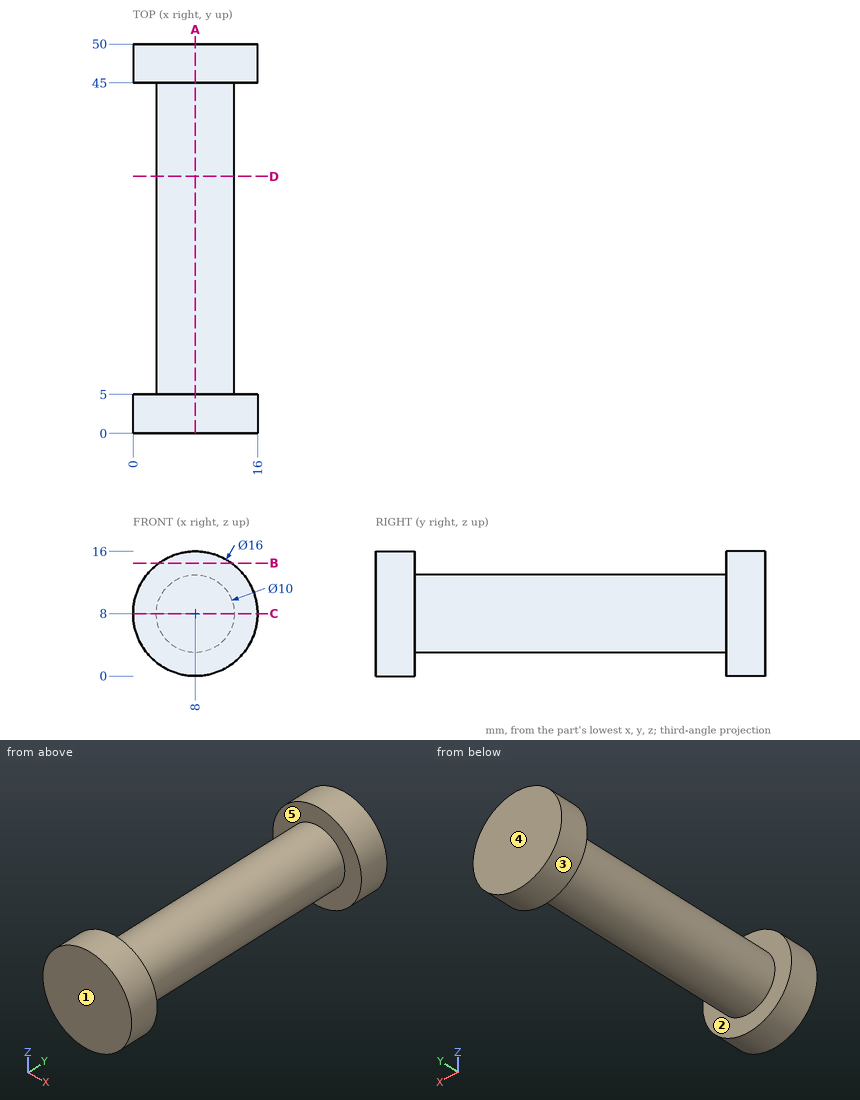
Input: dimensioned drawing with shaded views. Units: mm. Origin: part minimum x, y, z. A direction names the side the tool comes from. Give positions to 0.01 mm unless a question says otherwise; leave off trailing zeros. Loops run counter-clockwise (first coordinate to the right, second up) from the corner with the lowest first, then second, coordinate; pieces in that order, holes last. Notation, with made-up numbers: (84.5, 36) - (90.5, 36) arc R22 cw to (90.5, 61) - close; hole circle Ø6 at (86, -37). An arc over 180 degrees is marked (long way). Answer as CSV lines item,"result". Start each with the question number.
(1) Ray query, line 1 along Y through (x, z) = (15.5, 7); line 2 along X through (y, z) = (17, 12); line 3 along X through (y, z) = (44, 3.5). Return the intervals inside material, ascending. Write a range as [from, to].
(2) Section query C-C (z = 8). Output: boundary loops of the cut face in (x, y).
(3) Reachability of the marked faces 1 and 2 from +Z, -Z, +X, -X, +Y, -Y: full face, straight path, thin tool, end or side. Return the list, or none.
(4) Section query B-B (z = 14.5). Output: boundary loops of the cut face in (x, y).
(5) Section query D-D (y = 33). Output: boundary loops of the cut face in (x, z), and give its area (3 significant figures).
(6) Mould query, pull axis Y, two halves, no side actions, for the marked faces 3, 4 and 5. Classes: +Y half, -Y half, draft (parallel to the pull), parting line (faces both ways), or undercut.
(7) Section query A-A (x = 8). Output: boundary loops of the cut face in (y, z), and give its area (3 significant figures).
(8) Pin query (flat end, axial travel): P1, Ø1, axis at y = 33, z = 12.5, coming from the -X side; P2, Ø6, axis at x = 3, z = 9.5, coming from the -Y side; P3, Ø8, axis at x = 9, y = 36.5, coming from the -Z side; P4, Ø5, axis at y = 38, z = 2.5, coming from the -X side. Return the tip coordinate at first contact, or that it passes through.
Worked answers:
1,line 1,"y = [0, 5], [45, 50]"
1,line 2,"x = [5, 11]"
1,line 3,"x = [5.82, 10.18]"
2,outline,"(0, 0) - (16, 0) - (16, 5) - (13, 5) - (13, 45) - (16, 45) - (16, 50) - (0, 50) - (0, 45) - (3, 45) - (3, 5) - (0, 5) - close"
3,face 1,"+Z, -Z, +X, -X, -Y"
3,face 2,"none"
4,outline,"(3.34, 0) - (12.66, 0) - (12.66, 5) - (3.34, 5) - close; (3.34, 45) - (12.66, 45) - (12.66, 50) - (3.34, 50) - close"
5,outline,"circle Ø10 at (8, 8)"
5,area,"78.5 mm^2"
6,face 3,"draft"
6,face 4,"+Y half"
6,face 5,"undercut"
7,outline,"(0, 0) - (5, 0) - (5, 3) - (45, 3) - (45, 0) - (50, 0) - (50, 16) - (45, 16) - (45, 13) - (5, 13) - (5, 16) - (0, 16) - close"
7,area,"560 mm^2"
8,P1,"stops at x = 5"
8,P2,"stops at y = 0"
8,P3,"stops at z = 3"
8,P4,"stops at x = 4"
